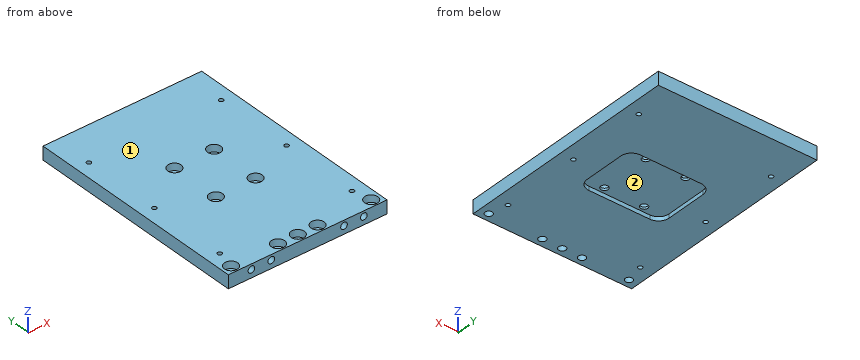
from build123d import *

# Parameters (mm, degrees)
SKETCH1_W                                           = 120
SKETCH1_H                                           = 170
BOSS_EXTRUDE1_DEPTH                                 = 5
M6_TAPPED_HOLE1_D                                   = 5
M6_TAPPED_HOLE1_DEPTH                               = 11.497848452
M6_TAPPED_HOLE1_TIP                                 = 1.502151548
CBORE_FOR_M5_HEX_SOCKET_HEAD_CAP_SCREW3_D           = 5.5
CBORE_FOR_M5_HEX_SOCKET_HEAD_CAP_SCREW3_DEPTH       = 20
CBORE_FOR_M5_HEX_SOCKET_HEAD_CAP_SCREW3_CBORE_D     = 10
CBORE_FOR_M5_HEX_SOCKET_HEAD_CAP_SCREW3_CBORE_DEPTH = 5.4
M4_TAPPED_HOLE1_D                                   = 3.3
CBORE_FOR_M5_HEX_SOCKET_HEAD_CAP_SCREW2_D           = 5.5
CBORE_FOR_M5_HEX_SOCKET_HEAD_CAP_SCREW2_CBORE_D     = 10
CBORE_FOR_M5_HEX_SOCKET_HEAD_CAP_SCREW2_CBORE_DEPTH = 5.4
CUT_EXTRUDE1_DEPTH                                  = 3


with BuildPart() as part:
    # Sketch1 → Boss-Extrude1 (new, symmetric)
    with BuildSketch(Plane.XY):
        Rectangle(SKETCH1_W, SKETCH1_H)
    extrude(amount=BOSS_EXTRUDE1_DEPTH, both=True)

    # M6 Tapped Hole1
    with Locations(Plane(origin=(0, -85, 0), x_dir=(-1, 0, 0), z_dir=(0, -1, 0))):
        with Locations((-42.5, -1), (-27.5, -1), (27.5, -1), (42.5, -1)):
            Hole(M6_TAPPED_HOLE1_D / 2, depth=M6_TAPPED_HOLE1_DEPTH)
            with Locations((0, 0, -(M6_TAPPED_HOLE1_DEPTH + M6_TAPPED_HOLE1_TIP / 2))):  # 118° drill point
                Cone(0, M6_TAPPED_HOLE1_D / 2, M6_TAPPED_HOLE1_TIP, mode=Mode.SUBTRACT)

    # CBORE for M5 Hex Socket Head Cap Screw3
    with Locations(Plane.XY.offset(5)):
        with Locations((53, -79), (12.5, -79), (-2.5, -79), (-17.5, -79), (-53, -79)):
            CounterBoreHole(CBORE_FOR_M5_HEX_SOCKET_HEAD_CAP_SCREW3_D / 2, CBORE_FOR_M5_HEX_SOCKET_HEAD_CAP_SCREW3_CBORE_D / 2, CBORE_FOR_M5_HEX_SOCKET_HEAD_CAP_SCREW3_CBORE_DEPTH, depth=CBORE_FOR_M5_HEX_SOCKET_HEAD_CAP_SCREW3_DEPTH)

    # M4 Tapped Hole1 (through all)
    with Locations(Plane(origin=(0, 0, -5), x_dir=(-1, 0, 0), z_dir=(0, 0, -1))):
        with Locations((50, -65), (50, -5), (50, 55), (-50, 55), (-50, -5), (-50, -65)):
            Hole(M4_TAPPED_HOLE1_D / 2)

    # CBORE for M5 Hex Socket Head Cap Screw2 (through all)
    with Locations(Plane.XY.offset(5)):
        with Locations((-15, 19), (15, 19), (15, -19), (-15, -19)):
            CounterBoreHole(CBORE_FOR_M5_HEX_SOCKET_HEAD_CAP_SCREW2_D / 2, CBORE_FOR_M5_HEX_SOCKET_HEAD_CAP_SCREW2_CBORE_D / 2, CBORE_FOR_M5_HEX_SOCKET_HEAD_CAP_SCREW2_CBORE_DEPTH)

    # Sketch35 → Cut-Extrude1 (cut)
    with BuildSketch(Plane(origin=(0, 0, -5), x_dir=(-1, 0, 0), z_dir=(0, 0, -1))):
        with BuildLine():
            Line((-23, 23.5), (23, 23.5))
            ThreePointArc((23, 23.5), (28.656854249, 21.156854249), (31, 15.5))
            Line((31, 15.5), (31, -15.5))
            ThreePointArc((31, -15.5), (28.656854249, -21.156854249), (23, -23.5))
            Line((23, -23.5), (-23, -23.5))
            ThreePointArc((-23, -23.5), (-28.656854249, -21.156854249), (-31, -15.5))
            Line((-31, -15.5), (-31, 15.5))
            ThreePointArc((-31, 15.5), (-28.656854249, 21.156854249), (-23, 23.5))
        make_face()
    extrude(amount=-CUT_EXTRUDE1_DEPTH, mode=Mode.SUBTRACT)


solid = part.part
Here's how the part is built. I have some questions about the finished solid (model axes, mm). Face numbers are marked on the shaded views. Round coordinates to 2 decimals unless told otherwise and drop trailing zeros. Order: outer loops, then holes, each group sorted by start corner. A loop starts at its lowest first (then second) coordinate and runs counter-clockwise, first axis right, second up. Notation, with made-up numbers: M -14,-24.5 L 1,-24.5 A8 ccw 1,-11.5 Z; hole C 16.5,7 d7. An arc over 180 degrees is marked long. Return JSON: item names as keys, results as strings. Group by question number.
1. If we section it at B-B on y = -19: List the corners of the cut face in (x, z) for me, then the cut area to 3 significant figures.
2. Please list where these lines run through material, in increasing order: probe 1 along X at (y, z) = (-65, -0.5); probe 2 along Y at (x, z) = (-53, 3.5); probe 3 along Y at (x, z) = (15, -1.35).
3. If we section it at C-C on y = -79: State how many separate pieces and enclosed holes the cut face has, then the cut area to 3 significant figures.
4. If we section it at A-A on x = -2.5: List the corners of the cut face in (y, z) for me, then the cut area to 3 significant figures.
5. I'm going to push flat-ended pins straight in: pin 1 Ø5 at (x, y) = (13, -77) entering from +Z; pin 2 Ø3 at (x, y) = (-50, -65) entering from -Z; pin 3 Ø8 at (x, y) = (-17.5, -79) entering from -Z; pin 4 Ø6.5 at (x, y) = (15, -19) entering from -Z. Where does each tip first touch, or does it pass through?
6. If we mould it in two halves opening along X, with no side actions, what happens to the marked faces 1 and 2? For each: pulls with the +X half, pulls with the -X half, needs draft (parallel to the pull), parting line crosses it, or undercut.
Reply:
{
 "1": {"outline": "M -60,-5 L -30.19,-5 L -30.19,-2 L -17.75,-2 L -17.75,-0.4 L -20,-0.4 L -20,5 L -60,5 Z; M -12.25,-2 L 12.25,-2 L 12.25,-0.4 L 10,-0.4 L 10,5 L -10,5 L -10,-0.4 L -12.25,-0.4 Z; M 17.75,-2 L 30.19,-2 L 30.19,-5 L 60,-5 L 60,5 L 20,5 L 20,-0.4 L 17.75,-0.4 Z", "area": "893 mm^2"},
 "2": {"probe 1": "-60 to -51.65, -48.35 to 48.35, 51.65 to 60", "probe 2": "-85 to -84, -74 to 85", "probe 3": "-85 to -80.15, -77.85 to -21.75, -16.25 to 16.25, 21.75 to 85"},
 "3": {"separate pieces": "6", "enclosed holes": "4", "area": "725 mm^2"},
 "4": {"outline": "M -85,-5 L -81.75,-5 L -81.75,-0.4 L -84,-0.4 L -84,5 L -85,5 Z; M -76.25,-5 L -23.5,-5 L -23.5,-2 L 23.5,-2 L 23.5,-5 L 85,-5 L 85,5 L -74,5 L -74,-0.4 L -76.25,-0.4 Z", "area": "1,480 mm^2"},
 "5": {"pin 1": "z = -0.4", "pin 2": "through", "pin 3": "z = -5", "pin 4": "z = -2"},
 "6": {"face 1": "needs draft", "face 2": "undercut"}
}
